from build123d import *

# Parameters (mm, degrees)
SKETCH1_R           = 11.5
BOSS_EXTRUDE1_DEPTH = 4
SKETCH2_R           = 2.25
CUT_EXTRUDE1_DEPTH  = 5
CHAMFER1_SIZE       = 2.5
CHAMFER1_SIZE2      = 3.087242891


with BuildPart() as part:
    # Sketch1 → Boss-Extrude1 (new body)
    with BuildSketch(Plane(origin=(0, 0, 0), x_dir=(1, 0, 0), z_dir=(0, 1, 0))):
        Circle(SKETCH1_R)
    extrude(amount=BOSS_EXTRUDE1_DEPTH)

    # Sketch2 → Cut-Extrude1 (cut, through all)
    with BuildSketch(Plane(origin=(0, 4, 0), x_dir=(1, 0, 0), z_dir=(0, 1, 0))):
        Circle(SKETCH2_R)
    extrude(amount=-CUT_EXTRUDE1_DEPTH, mode=Mode.SUBTRACT)

    # Chamfer1
    chamfer1_edges = [part.edges().sort_by_distance(p)[0] for p in [
        (-2.25, 0, 0),
    ]]
    chamfer1_side = [part.faces().sort_by_distance(p)[0] for p in [
        (-11.174730881, 0, 0),
    ]]
    chamfer(chamfer1_edges, length=CHAMFER1_SIZE, length2=CHAMFER1_SIZE2, reference=chamfer1_side[0])


solid = part.part
Verification items for the finished model (mm, model axes). Give positions to 0.01 mm unless a question says otherwise; leave off trailing zeros. Order: outer loops, then holes, each group sorted by start corner. A loop starts at its lowest first (then second) coordinate and runs counter-clockwise, first axis right, second up. Notation, with made-up numbers: M 71,-40 L 95,-40 A29 ccw 95,-13 Z; hole C 78.25,19 d1. An arc over 180 degrees is marked long. Use one line per item in the form item = value. Start each with the question number.
Q1. Section check D-D (z = -8.5). Enter the section's corners in (x, y).
Q2. Section check B-B (z = 0). Enter the section's corners in (x, y).
Q3. Mould release check, pull along X, two halves, no side actions. Record for faces 1 (the conical face through (-0.514, 2.937, 2.315)), 2 (the flat face through (-0.2, 4, 2.4)), 3 (the cylindrical face through (-1.5, 2, -11.4)): +X half, -X half, draft (parallel to the pull), parting line (faces both ways), or undercut.
Q4. Scan lines: line 1 along X through (y, z) = (3.4, 0); line 2 along X through (y, z) = (1.8, 3). Record each from-to range of solid material in increasing order. Write a range as [from, to].
Q5. Section check A-A (x = 0). Enter the section's corners in (y, z).
Q6. Go/stop test with flat-tipped pins: pin 1 Ø1 at (x, y) = (8.5, 0.5) entering from +Z; pin 2 Ø5 at (x, z) = (0, 0) entering from -Y. Record where each tip stops, or that it passes through.
Q7. Section check C-C (y = 3.5). Enter the section's corners in (x, z), then the cut area to 3 significant figures.
Evaluation:
q1.outline = M -7.75,0 L 7.75,0 L 7.75,4 L -7.75,4 Z
q2.outline = M -11.5,0 L -4.75,0 L -2.25,3.09 L -2.25,4 L -11.5,4 Z; M 2.25,3.09 L 4.75,0 L 11.5,0 L 11.5,4 L 2.25,4 Z
q3.face_1 = undercut
q3.face_2 = draft
q3.face_3 = parting line
q4.line_1 = [-11.5, -2.25], [2.25, 11.5]
q4.line_2 = [-11.1, -1.36], [1.36, 11.1]
q5.outline = M 0,-11.5 L 4,-11.5 L 4,-2.25 L 3.09,-2.25 L 0,-4.75 Z; M 0,4.75 L 3.09,2.25 L 4,2.25 L 4,11.5 L 0,11.5 Z
q6.pin_1 = 8.26
q6.pin_2 = 2.78
q7.outline = C 0,0 d23; hole C 0,0 d4.5
q7.area = 400 mm2
